from build123d import *

# Parameters (mm, degrees)
F0_W         = 6.35
F0_H         = 6.35
F0_W_2       = 4.572
F0_H_2       = 4.572
F1_DEPTH     = 50.8
F3_T1_DEPTH  = 4.572
F3_T3_DEPTH  = 4.572
F3_T9_DEPTH  = 7.8380373947
F3_T15_DEPTH = 7.8380373947
F3_T24_DEPTH = 7.8380373947
F3_T30_DEPTH = 7.8380373947
F3_T39_DEPTH = 7.8380373947
F3_T45_DEPTH = 7.8380373947
F3_T54_DEPTH = 7.8380373947
F3_T60_DEPTH = 7.8380373947
F4_T1_DEPTH  = 12.8820747894
F4_T3_DEPTH  = 12.8820747894
F5_DEPTH     = 3.175
F6_T1_DEPTH  = 6.35
F6_T3_DEPTH  = 6.35
F6_T5_DEPTH  = 6.35
F6_T7_DEPTH  = 6.35
F6_T9_DEPTH  = 32.1381754825
F6_T11_DEPTH = 32.1381754825
F6_T13_DEPTH = 32.1381754825
F6_T15_DEPTH = 32.1381754825


# Not quite as in the source:
# - a fillet or chamfer that OpenCascade refuses, or shapes differently, is made with other operations: its cross-section is extruded or revolved along the edge and cut away or added


with BuildPart() as f1:
    # F0 (on Top) → F1 (new body, symmetric)
    with BuildSketch(Plane.XY):
        Rectangle(F0_W, F0_H)
        Rectangle(F0_W_2, F0_H_2, mode=Mode.SUBTRACT)
    extrude(amount=F1_DEPTH, both=True)

    # F3: chamfer of 1.27 on 4 edges, made by hand

    # F3_s2 → F3_t1 (cut)
    with BuildSketch(Plane.YZ.offset(-2.286)):
        Polygon((3.556, 50.8), (2.286, 49.53), (2.286, 50.8), align=None)
        Polygon((-3.556, 50.8), (-2.286, 49.53), (-2.286, 50.8), align=None)
    extrude(amount=F3_T1_DEPTH, mode=Mode.SUBTRACT)

    # F3_s4 → F3_t3 (cut)
    with BuildSketch(Plane.XZ.offset(-2.286)):
        Polygon((-3.556, 50.8), (-2.286, 49.53), (-2.286, 50.8), align=None)
        Polygon((3.556, 50.8), (2.286, 49.53), (2.286, 50.8), align=None)
    extrude(amount=F3_T3_DEPTH, mode=Mode.SUBTRACT)


with BuildPart() as f3_tool7:
    # F3_s8 → F3_t9 (new body)
    with BuildSketch(Plane.YZ.offset(-5.5520373947)):
        Polygon((3.556, 50.8), (2.286, 49.53), (2.286, 50.8), align=None)
    extrude(amount=F3_T9_DEPTH)

    split(bisect_by=Plane.YZ.offset(-3.175), keep=Keep.TOP)

    split(bisect_by=Plane.YZ.offset(-2.286), keep=Keep.BOTTOM)

    split(bisect_by=Plane.XZ.offset(-3.175), keep=Keep.TOP)


with BuildPart() as f3_tool13:
    # F3_s14 → F3_t15 (new body)
    with BuildSketch(Plane.XZ.offset(2.286)):
        Polygon((-3.556, 50.8), (-2.286, 49.53), (-2.286, 50.8), align=None)
    extrude(amount=-F3_T15_DEPTH)

    split(bisect_by=Plane.YZ.offset(-3.175), keep=Keep.TOP)

    split(bisect_by=Plane.XZ.offset(-2.286), keep=Keep.BOTTOM)

    split(bisect_by=Plane.XZ.offset(-3.175), keep=Keep.TOP)


with BuildPart() as f3_tool7_1:
    add(f3_tool7.part)

    # F3_t19: intersect F3_tool13
    add(f3_tool13.part, mode=Mode.INTERSECT)


with BuildPart() as f1_1:
    add(f1.part)

    # F3_t5: cut F3_tool7
    add(f3_tool7_1.part, mode=Mode.SUBTRACT)


with BuildPart() as f3_tool22:
    # F3_s23 → F3_t24 (new body)
    with BuildSketch(Plane.YZ.offset(-2.286)):
        Polygon((3.556, 50.8), (2.286, 49.53), (2.286, 50.8), align=None)
    extrude(amount=F3_T24_DEPTH)

    split(bisect_by=Plane.YZ.offset(3.175), keep=Keep.BOTTOM)

    split(bisect_by=Plane.YZ.offset(2.286), keep=Keep.TOP)

    split(bisect_by=Plane.XZ.offset(-3.175), keep=Keep.TOP)


with BuildPart() as f3_tool28:
    # F3_s29 → F3_t30 (new body)
    with BuildSketch(Plane.XZ.offset(-5.5520373947)):
        Polygon((3.556, 50.8), (2.286, 49.53), (2.286, 50.8), align=None)
    extrude(amount=F3_T30_DEPTH)

    split(bisect_by=Plane.YZ.offset(3.175), keep=Keep.BOTTOM)

    split(bisect_by=Plane.XZ.offset(-2.286), keep=Keep.BOTTOM)

    split(bisect_by=Plane.XZ.offset(-3.175), keep=Keep.TOP)


with BuildPart() as f3_tool22_1:
    add(f3_tool22.part)

    # F3_t34: intersect F3_tool28
    add(f3_tool28.part, mode=Mode.INTERSECT)


with BuildPart() as f1_2:
    add(f1_1.part)

    # F3_t20: cut F3_tool22
    add(f3_tool22_1.part, mode=Mode.SUBTRACT)


with BuildPart() as f3_tool37:
    # F3_s38 → F3_t39 (new body)
    with BuildSketch(Plane.YZ.offset(2.286)):
        Polygon((-3.556, 50.8), (-2.286, 49.53), (-2.286, 50.8), align=None)
    extrude(amount=-F3_T39_DEPTH)

    split(bisect_by=Plane.XZ.offset(3.175), keep=Keep.BOTTOM)

    split(bisect_by=Plane.YZ.offset(-3.175), keep=Keep.TOP)

    split(bisect_by=Plane.YZ.offset(-2.286), keep=Keep.BOTTOM)


with BuildPart() as f3_tool43:
    # F3_s44 → F3_t45 (new body)
    with BuildSketch(Plane.XZ.offset(5.5520373947)):
        Polygon((-3.556, 50.8), (-2.286, 49.53), (-2.286, 50.8), align=None)
    extrude(amount=-F3_T45_DEPTH)

    split(bisect_by=Plane.XZ.offset(3.175), keep=Keep.BOTTOM)

    split(bisect_by=Plane.YZ.offset(-3.175), keep=Keep.TOP)

    split(bisect_by=Plane.XZ.offset(2.286), keep=Keep.TOP)


with BuildPart() as f3_tool37_1:
    add(f3_tool37.part)

    # F3_t49: intersect F3_tool43
    add(f3_tool43.part, mode=Mode.INTERSECT)


with BuildPart() as f1_3:
    add(f1_2.part)

    # F3_t35: cut F3_tool37
    add(f3_tool37_1.part, mode=Mode.SUBTRACT)


with BuildPart() as f3_tool52:
    # F3_s53 → F3_t54 (new body)
    with BuildSketch(Plane.XZ.offset(-2.286)):
        Polygon((3.556, 50.8), (2.286, 49.53), (2.286, 50.8), align=None)
    extrude(amount=F3_T54_DEPTH)

    split(bisect_by=Plane.YZ.offset(3.175), keep=Keep.BOTTOM)

    split(bisect_by=Plane.XZ.offset(3.175), keep=Keep.BOTTOM)

    split(bisect_by=Plane.XZ.offset(2.286), keep=Keep.TOP)


with BuildPart() as f3_tool58:
    # F3_s59 → F3_t60 (new body)
    with BuildSketch(Plane.YZ.offset(5.5520373947)):
        Polygon((-3.556, 50.8), (-2.286, 49.53), (-2.286, 50.8), align=None)
    extrude(amount=-F3_T60_DEPTH)

    split(bisect_by=Plane.YZ.offset(3.175), keep=Keep.BOTTOM)

    split(bisect_by=Plane.XZ.offset(3.175), keep=Keep.BOTTOM)

    split(bisect_by=Plane.YZ.offset(2.286), keep=Keep.TOP)


with BuildPart() as f3_tool52_1:
    add(f3_tool52.part)

    # F3_t64: intersect F3_tool58
    add(f3_tool58.part, mode=Mode.INTERSECT)


with BuildPart() as f1_4:
    add(f1_3.part)

    # F3_t50: cut F3_tool52
    add(f3_tool52_1.part, mode=Mode.SUBTRACT)

    # F4: chamfer of 1.27 on 4 edges, made by hand

    # F4_s2 → F4_t1 (cut)
    with BuildSketch(Plane.XZ.offset(-6.4410373947)):
        Polygon((3.175, -49.53), (1.905, -50.8), (3.175, -50.8), align=None)
        Polygon((-3.175, -49.53), (-1.905, -50.8), (-3.175, -50.8), align=None)
    extrude(amount=F4_T1_DEPTH, mode=Mode.SUBTRACT)

    # F4_s4 → F4_t3 (cut)
    with BuildSketch(Plane.YZ.offset(-6.4410373947)):
        Polygon((-1.905, -50.8), (-3.175, -49.53), (-3.175, -50.8), align=None)
        Polygon((3.175, -49.53), (1.905, -50.8), (3.175, -50.8), align=None)
    extrude(amount=F4_T3_DEPTH, mode=Mode.SUBTRACT)

    # F2 (on Right) → F5 (join, symmetric)
    with BuildSketch(Plane.YZ):
        Polygon((-19.1053829622, 41.8550837785), (-2.5904842187, 18.636116758), (-2.3452136666, 21.0888255388), (-16.897945432, 41.8550837785), align=None)
        Polygon((-19.3506535143, -16.5116898715), (-2.8357547708, -39.7306568921), (-2.5904842187, -37.2779481113), (-17.1432159841, -16.5116898715), align=None)
        Polygon((2.5904842187, 18.636116758), (19.1053829622, 41.8550837785), (16.897945432, 41.8550837785), (2.3452136666, 21.0888255388), align=None)
        Polygon((17.1432159841, -16.5116898715), (2.5904842187, -37.2779481113), (2.8357547708, -39.7306568921), (19.3506535143, -16.5116898715), align=None)
    extrude(amount=F5_DEPTH, both=True)

    # F6: fillet of radius 5.08 on 8 edges, made by hand

    # F6_s2 → F6_t1 (join)
    with BuildSketch(Plane.YZ.offset(-3.175)):
        with BuildLine():
            ThreePointArc((-3.175, -40.8760570484), (-3.415789898, -39.3305973794), (-4.1153329089, -37.931646008))
            Line((-4.1153329089, -37.931646008), (-3.175, -39.2536982433))
            Line((-3.175, -39.2536982433), (-3.175, -40.8760570484))
        make_face()
    extrude(amount=F6_T1_DEPTH)

    # F6_s4 → F6_t3 (join)
    with BuildSketch(Plane.YZ.offset(-3.175)):
        with BuildLine():
            ThreePointArc((-4.1153329089, 20.7799634748), (-3.415789898, 19.3810121034), (-3.175, 17.8355524344))
            Line((-3.175, 17.8355524344), (-3.175, 19.4579112395))
            Line((-3.175, 19.4579112395), (-4.1153329089, 20.7799634748))
        make_face()
    extrude(amount=F6_T3_DEPTH)

    # F6_s6 → F6_t5 (join)
    with BuildSketch(Plane.YZ.offset(-3.175)):
        with BuildLine():
            ThreePointArc((3.175, 17.8355524344), (3.415789898, 19.3810121034), (4.1153329089, 20.7799634748))
            Line((4.1153329089, 20.7799634748), (3.175, 19.4579112395))
            Line((3.175, 19.4579112395), (3.175, 17.8355524344))
        make_face()
    extrude(amount=F6_T5_DEPTH)

    # F6_s8 → F6_t7 (join)
    with BuildSketch(Plane.YZ.offset(-3.175)):
        with BuildLine():
            ThreePointArc((3.175, -40.8760570484), (3.415789898, -39.3305973794), (4.1153329089, -37.931646008))
            Line((4.1153329089, -37.931646008), (3.175, -39.2536982433))
            Line((3.175, -39.2536982433), (3.175, -40.8760570484))
        make_face()
    extrude(amount=F6_T7_DEPTH)

    # F6_s10 → F6_t9 (cut)
    with BuildSketch(Plane.YZ.offset(-16.0690877412)):
        with BuildLine():
            ThreePointArc((-17.1432159841, -16.5116898715), (-17.2158715108, -18.6994178747), (-16.3612445142, -20.7146214221))
            Line((-16.3612445142, -20.7146214221), (-19.3506535143, -16.5116898715))
            Line((-19.3506535143, -16.5116898715), (-17.1432159841, -16.5116898715))
        make_face()
    extrude(amount=F6_T9_DEPTH, mode=Mode.SUBTRACT)

    # F6_s12 → F6_t11 (cut)
    with BuildSketch(Plane.YZ.offset(-16.0690877412)):
        with BuildLine():
            ThreePointArc((-16.1159739621, 37.6521522279), (-16.9706009587, 39.6673557754), (-16.897945432, 41.8550837785))
            Line((-16.897945432, 41.8550837785), (-19.1053829622, 41.8550837785))
            Line((-19.1053829622, 41.8550837785), (-16.1159739621, 37.6521522279))
        make_face()
    extrude(amount=F6_T11_DEPTH, mode=Mode.SUBTRACT)

    # F6_s14 → F6_t13 (cut)
    with BuildSketch(Plane.YZ.offset(-16.0690877412)):
        with BuildLine():
            ThreePointArc((16.897945432, 41.8550837785), (16.9706009587, 39.6673557754), (16.1159739621, 37.6521522279))
            Line((16.1159739621, 37.6521522279), (19.1053829622, 41.8550837785))
            Line((19.1053829622, 41.8550837785), (16.897945432, 41.8550837785))
        make_face()
    extrude(amount=F6_T13_DEPTH, mode=Mode.SUBTRACT)

    # F6_s16 → F6_t15 (cut)
    with BuildSketch(Plane.YZ.offset(-16.0690877412)):
        with BuildLine():
            ThreePointArc((17.1432159841, -16.5116898715), (17.2158715108, -18.6994178747), (16.3612445142, -20.7146214221))
            Line((16.3612445142, -20.7146214221), (19.3506535143, -16.5116898715))
            Line((19.3506535143, -16.5116898715), (17.1432159841, -16.5116898715))
        make_face()
    extrude(amount=F6_T15_DEPTH, mode=Mode.SUBTRACT)


solid = f1_4.part
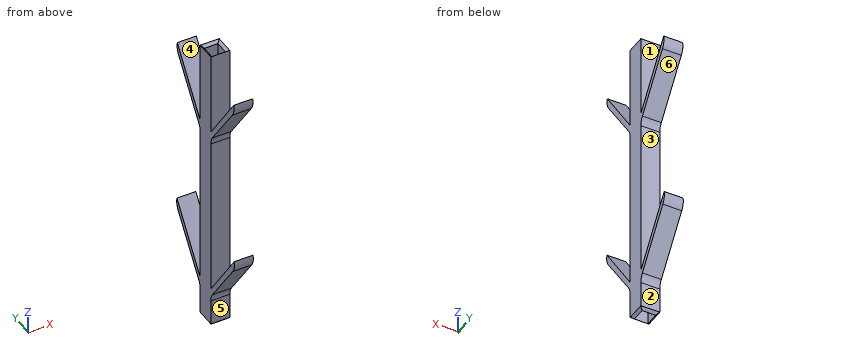
Can you work these out from the model? Positions are in its coordinate system, mm. Face numbers are marked on the shaded views. A direction names the side the tool comes from. Coordinates: 2 decimals unless noted, no trailing zeros. Loops run counter-clockwise (first coordinate to the right, second up) from the corner with the lowest first, then second, coordinate; pieces in that order, holes last. Notation, with made-up numbers: M 20.25,-0.5 L 50.25,-0.5 A18 ccw 50.25,4.5 Z; hole C -27.75,68.25 d1. An arc over 180 degrees is marked long. Answer as CSV lines item,"result". Start each with the question number.
1. Thinking about a two-plate mould opening in Y: for the marked faces 4, 5 and 6, which applies, +Y half, -Y half, draft (parallel to the pull), parting line (faces both ways), or undercut?
2. If I drill on probe 1 along X at (y, z) = (-2, 32.5) (3 decimals); probe 2 along Y at (x, z) = (1, -35.5) (3 decimals), over which ranges is the centre line in solid material (lowest first)? Write a range as [from, to].
3. For pin 1 Ø2 at (x, y) = (2, 13.5) entering from -Z; pin 2 Ø5 at (y, z) = (9.5, -19) entering from +X (1 decimal); pin 3 Ø1.9 at (x, z) = (-1.5, -47.5) entering from +Y (3 decimals); pin 4 Ø3 at (x, y) = (0, 12) entering from +Z, each with a flat end and sliding along its axis, tell me the tip position at first contact or that it passes through.
4. Suppose I cut it at A-A, the plane z = -22.5. List the corners of the cut face in (x, y) for me (3 decimals), plus the area to 3 significant figures.
5. For the marked faces 1, 2 and 3, which set-ups out of +Z, -Z, +X, -X, +Y, -Y let a thin tool reach every point of the face, with its end or its side?
6. Suppose I cut it at C-C, the plane z = -7. List the corners of the cut face in (x, y) for me (3 decimals), plus the area to 3 significant figures.
7. Suppose I cut it at D-D, the plane y = 10.5. List the corners of the cut face in (x, z) for me (3 decimals).
8. Suppose I cut it at B-B, the plane y = -8.5. List the corners of the cut face in (x, z) for me (1 decimal), plus the area to 3 significant figures.
Output:
1,face 4,"undercut"
1,face 5,"-Y half"
1,face 6,"+Y half"
2,probe 1,"x = [-3.175, -2.286], [2.286, 3.175]"
2,probe 2,"y = [-5.845, -3.836], [-3.175, -2.286], [2.286, 3.175], [3.836, 5.845]"
3,pin 1,"stops at z = -26.14"
3,pin 2,"passes through"
3,pin 3,"stops at y = 3.175"
3,pin 4,"stops at z = 37.01"
4,outline,"M -3.175,-15.091 L 3.175,-15.091 L 3.175,-12.947 L -3.175,-12.947 Z; M -3.175,-3.175 L 3.175,-3.175 L 3.175,3.175 L -3.175,3.175 Z; M -3.175,12.947 L 3.175,12.947 L 3.175,15.091 L -3.175,15.091 Z; hole M -2.286,-2.286 L 2.286,-2.286 L 2.286,2.286 L -2.286,2.286 Z"
4,area,"46.7 mm^2"
5,face 1,"+Z, +X, -X"
5,face 2,"-Z, +X, -X, +Y"
5,face 3,"+X, -X"
6,outline,"M -3.175,-3.175 L 3.175,-3.175 L 3.175,3.175 L -3.175,3.175 Z; hole M -2.286,-2.286 L 2.286,-2.286 L 2.286,2.286 L -2.286,2.286 Z"
6,area,"19.4 mm^2"
7,outline,"M -3.175,-28.955 L 3.175,-28.955 L 3.175,-25.991 L -3.175,-25.991 Z; M -3.175,29.756 L 3.175,29.756 L 3.175,32.725 L -3.175,32.725 Z"
8,outline,"M -3.2,-31.8 L 3.2,-31.8 L 3.2,-28.8 L -3.2,-28.8 Z; M -3.2,26.9 L 3.2,26.9 L 3.2,29.9 L -3.2,29.9 Z"
8,area,"37.1 mm^2"
